from build123d import *

# Parameters (mm, degrees)
F0_R     = 7.5
F0_R_2   = 4
F1_DEPTH = 12
F2_W     = 1
F2_H     = 1.1
F4_R     = 6.5
F4_R_2   = 5
F5_DEPTH = 0.5
F6_R     = 6.5
F6_R_2   = 5
F7_DEPTH = 0.5
F8_R     = 0.5


with BuildPart() as f1:
    # F0 (on Front) → F1 (new body, symmetric)
    with BuildSketch(Plane.XZ):
        Circle(F0_R)
        Circle(F0_R_2, mode=Mode.SUBTRACT)
    extrude(amount=F1_DEPTH, both=True)

    # F2 (on Top) → F3 (revolve, cut)
    with BuildSketch(Plane.XY):
        with Locations((-7.65, 8.2)):
            Rectangle(F2_W, F2_H)
        with Locations((-7.65, -8.2)):
            Rectangle(F2_W, F2_H)
    revolve(axis=Axis((0, 10.336502, 0), (0, 1, 0)), mode=Mode.SUBTRACT)

    # F4 (on face) → F5 (cut)
    with BuildSketch(Plane.XZ.offset(12)):
        Circle(F4_R)
        Circle(F4_R_2, mode=Mode.SUBTRACT)
    extrude(amount=-F5_DEPTH, mode=Mode.SUBTRACT)

    # F6 (on face) → F7 (cut)
    with BuildSketch(Plane(origin=(0, 12, 0), x_dir=(-1, 0, 0), z_dir=(0, 1, 0))):
        Circle(F6_R)
        Circle(F6_R_2, mode=Mode.SUBTRACT)
    extrude(amount=-F7_DEPTH, mode=Mode.SUBTRACT)

    # F8
    f8_edges = [f1.edges().sort_by_distance(p)[0] for p in [
        (-7.5, 12, 0),
        (-7.5, -12, 0),
    ]]
    fillet(f8_edges, radius=F8_R)


solid = f1.part
Design review of the part built by this model. Coordinates are the model's own, in mm. A direction names the side the tool comes from. Coordinates: 2 decimals unless noted, no trailing zeros. Loops run counter-clockwise (first coordinate to the right, second up) from the corner with the lowest first, then second, coordinate; pieces in that order, holes last. Notation, with made-up numbers: M 27.5,36 L 61.5,36 A18 ccw 61.5,52 Z; hole C 32,51 d10. An arc over 180 degrees is marked long. Use one line per item in the form item = value.
(1) Draft analysis for pull direction Y (two halves, no side actions). For faces 1 (the face through (2, -11.5, -5)), 2 (the face through (-2, 11.5, -5)), 3 (the face through (-7.493, 10.106, 0.33)), 4 (the face through (0.93, -8.19, 7.09)), state which applies: pulls with the +Y half, pulls with the -Y half, needs draft (parallel to the pull), parting line crosses it, or undercut.
Return value:
face_1 = pulls with the -Y half
face_2 = pulls with the +Y half
face_3 = needs draft
face_4 = undercut
(2) Consider section A-A (y = -8). Write out the cut boundary in (x, z).
Return value:
outline = C 0,0 d14.3; hole C 0,0 d8
(3) Clearance check with flat-ended pins moving along their axes: P1, Ø4, axis at y = 2.5, z = -5, coming from the +X side; P2, Ø5, axis at x = 0, z = 0, coming from the -Y side; P3, Ø3, axis at x = -5.5, y = -4, coming from the -Z side. State where each tip first meets the part, or that it passes through.
Return value:
P1 = 6.87
P2 = through
P3 = -6.34
(4) For line 1 along Z through (x, y) = (0, 5.25); line 2 along Z through (x, y) = (0, 11.9); line 3 along Y through (x, z) = (5.5, -3), list the stretches that pass through material, from the lowest coordinate up. Write a range as from..to.
Return value:
line_1 = -7.5..-4, 4..7.5
line_2 = -7.3..-6.5, -5..-4, 4..5, 6.5..7.3
line_3 = -11.5..11.5
(5) For faces 5 (the face through (-5.158, -11.754, -3.955)), 6 (the face through (5.158, 11.754, -3.955)), 7 (the face through (-0.867, 0.168, -3.905)), list the 3-axis set-ups (+Z, -Z, +X, -X, +Y, -Y) from which the entire face can be reached by the end or side of a thin tool; tool diameter is ignored.
Return value:
face_5 = -Y
face_6 = +Y
face_7 = +Y, -Y
(6) Consider section B-B (y = 0.25). Write out the cut boundary in (x, z).
Return value:
outline = C 0,0 d15; hole C 0,0 d8
